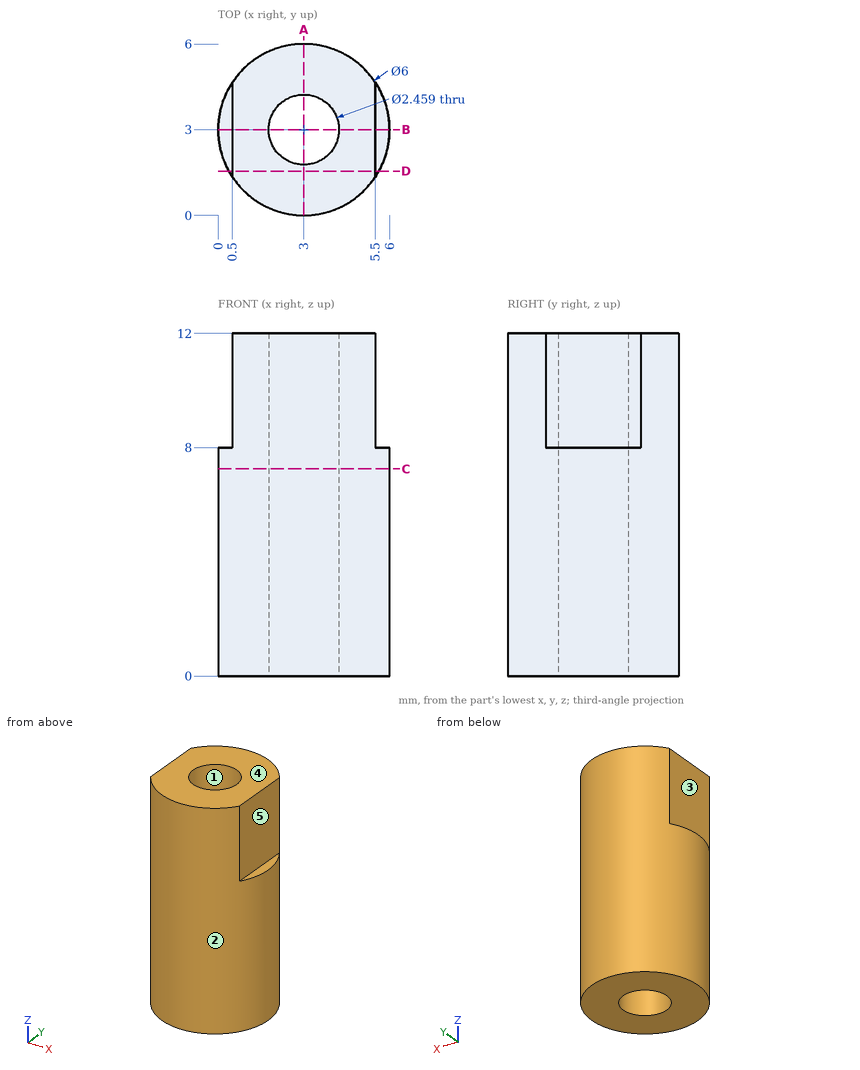
The drawing under review shows one solid part. Ordinate dimensions are in mm from its lowest x, y, z. A direction names the side the tool comes from. Round coordinates to 2 decimals unless told otherwise and drop trailing zeros. Write each loop counter-clockwise with the first axis right and the second up, starting at its lowest first coordinate (ties: lowest second). Pieces come first, ordered by that corner, then holes. Notation, with made-up numbers: (-33, 12) -> (-7, 12) arc R37 ccw to (-7, 48) -> close; hole circle Ø10 at (63.25, 83). An arc over 180 degrees is marked (long way). Put each result on its own line as item: value.
Q1. Machinability: for the marked faces 4 and 5, which of the approach directions +Z, -Z, +X, -X, +Y, -Y give a long, thin tool a straight path to every point of the face, cutting with its end or side? Answer none if there is none.
Determined:
face 4: +Z, +X, -X, +Y, -Y
face 5: +Z, +X, +Y, -Y
Q2. To check wall thickness, follow L1, parallel to X at y = 3, z = 7.75; L2, parallel to Z at x = 5.55, y = 3.15; L3, parallel to Y at x = 2.35, z = 1.75. State the ranges of each line that lie inside material, in increasing order. Write a range as [from, to].
Determined:
L1: x = [0, 1.77], [4.23, 6]
L2: z = [0, 8]
L3: y = [0.07, 1.96], [4.04, 5.93]
Q3. Consider section D-D on y = 1.55. State the section outline as (x, z) points, and give its area (3 significant figures).
Determined:
outline: (0.37, 0) -> (5.63, 0) -> (5.63, 8) -> (5.5, 8) -> (5.5, 12) -> (0.5, 12) -> (0.5, 8) -> (0.37, 8) -> close
area: 62.0 mm^2
Q4. Consider section C-C on z = 7.25. State the section outline as (x, y) points, and give its area (3 significant figures).
Determined:
outline: circle Ø6 at (3, 3); hole circle Ø2.46 at (3, 3)
area: 23.5 mm^2
Q5. Consider section A-A on x = 3. State the section outline as (y, z) points.
Determined:
outline: (0, 0) -> (1.77, 0) -> (1.77, 12) -> (0, 12) -> close; (4.23, 0) -> (6, 0) -> (6, 12) -> (4.23, 12) -> close
Q6. Clearance check with flat-ended pins moving along their axes: pin 1 Ø1 at (y, z) = (5, 6.5) entering from +X; pin 2 Ø3 at (y, z) = (5, 2.5) entering from -X; pin 3 Ø3.5 at (y, z) = (3, 10) entering from +X. State where each tip first meets the part, or that it passes through.
Determined:
pin 1: stops at x = 5.6
pin 2: stops at x = 0.04
pin 3: stops at x = 5.5
Q7. Consider section B-B on y = 3. State the section outline as (x, z) points, and give its area (3 significant figures).
Determined:
outline: (0, 0) -> (1.77, 0) -> (1.77, 12) -> (0.5, 12) -> (0.5, 8) -> (0, 8) -> close; (4.23, 0) -> (6, 0) -> (6, 8) -> (5.5, 8) -> (5.5, 12) -> (4.23, 12) -> close
area: 38.5 mm^2
Q8. The part is to be moulded in two halves that separate along Y. For the marked faces 1, 2 and 3, say which applies: released by +Y, released by -Y, zero draft, split by the parting line, or undercut.
Determined:
face 1: undercut
face 2: split by the parting line
face 3: zero draft
